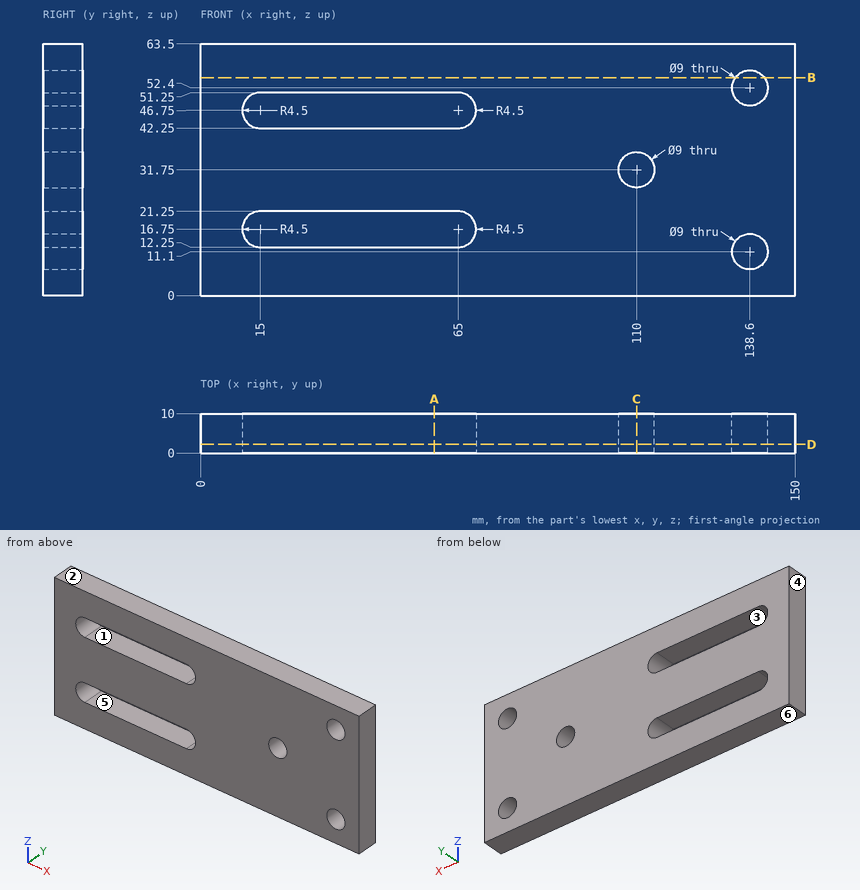
Here's the drawing with two shaded views (mm, measured from the low corner). I have some questions. A direction names the side the tool comes from. Round coordinates to 2 decimals unless told otherwise and drop trailing zeros. Order: outer loops, then holes, each group sorted by start corner. A loop starts at its lowest first (then second) coordinate and runs counter-clockwise, first axis right, second up. Notation, with made-up numbers: (83, 17) -> (126, 17) arc R26 ccw to (126, 42) -> close; hole circle Ø11 at (75.25, -3.5). An arc over 180 degrees is marked (long way). Use a Markdown table: item, result. Add a question column.
(1) Suppose I cut it at C-C, the plane x = 110. Please give me the cut outline in (y, z), and give its area (3 significant figures).
(2) If we mould it in two halves opening along X, with no side actions, what happens to the marked faces 1, 2, 3 and 4? For each: released by +X, released by -X, zero draft, split by the parting line, or undercut.
(3) For the marked faces 5 and 6, which set-ups out of +Z, -Z, +X, -X, +Y, -Y let a thin tool reach every point of the face, with its end or its side?
(4) Suppose I cut it at A-A, the plane x = 59. Please give me the cut outline in (y, z).
(5) Suppose I cut it at D-D, the plane y = 2.25. Please give me the cut outline in (x, z), and give its area (3 significant figures).
(6) Suppose I cut it at B-B, the plane z = 55. Please give me the cut outline in (x, y), and give its area (3 significant figures).
(7) For pin 1 Ø5 at (x, y) = (47.5, 6) entering from -Z; pin 2 Ø8 at (x, z) = (110, 31.75) entering from +Y, each with a flat end and sliding along its axis, tell me the tip position at first contact or that it passes through.
(8) I need wall thicknesses on line 1 along Z through (x, y) = (138.6, 6.25); line 2 along Z through (x, y) = (28.5, 8); line 3 along X through (y, z) = (9.5, 48.5) (3 decimals). Which ranges of each line are inside material? Lowest first, please.
Verdict:
| question | item | result |
|---|---|---|
| 1 | outline | (0, 0) -> (10, 0) -> (10, 27.25) -> (0, 27.25) -> close; (0, 36.25) -> (10, 36.25) -> (10, 63.5) -> (0, 63.5) -> close |
| 1 | area | 545 mm2 |
| 2 | face 1 | undercut |
| 2 | face 2 | zero draft |
| 2 | face 3 | undercut |
| 2 | face 4 | released by -X |
| 3 | face 5 | +Y, -Y |
| 3 | face 6 | -Z, +X, -X, +Y, -Y |
| 4 | outline | (0, 0) -> (10, 0) -> (10, 12.25) -> (0, 12.25) -> close; (0, 21.25) -> (10, 21.25) -> (10, 42.25) -> (0, 42.25) -> close; (0, 51.25) -> (10, 51.25) -> (10, 63.5) -> (0, 63.5) -> close |
| 5 | outline | (0, 0) -> (150, 0) -> (150, 63.5) -> (0, 63.5) -> close; hole (15, 12.25) -> (65, 12.25) arc R4.5 ccw to (65, 21.25) -> (15, 21.25) arc R4.5 ccw to start; hole (15, 42.25) -> (65, 42.25) arc R4.5 ccw to (65, 51.25) -> (15, 51.25) arc R4.5 ccw to start; hole circle Ø9 at (110, 31.75); hole circle Ø9 at (138.6, 11.1); hole circle Ø9 at (138.6, 52.4) |
| 5 | area | 8,310 mm2 |
| 6 | outline | (0, 0) -> (134.93, 0) -> (134.93, 10) -> (0, 10) -> close; (142.27, 0) -> (150, 0) -> (150, 10) -> (142.27, 10) -> close |
| 6 | area | 1,430 mm2 |
| 7 | pin 1 | z = 0 |
| 7 | pin 2 | through |
| 8 | line 1 | 0 to 6.6, 15.6 to 47.9, 56.9 to 63.5 |
| 8 | line 2 | 0 to 12.25, 21.25 to 42.25, 51.25 to 63.5 |
| 8 | line 3 | 0 to 10.854, 69.146 to 136.355, 140.845 to 150 |
